```python
from build123d import *

# Parameters (mm, degrees)
SKETCH1_R           = 9.525
BOSS_EXTRUDE1_DEPTH = 6.35
CUT_EXTRUDE1_START  = -6.35
CUT_EXTRUDE1_DEPTH  = 6.35
CUT_EXTRUDE2_START  = -6.35
CUT_EXTRUDE2_DEPTH  = 6.35
SKETCH4_R           = 1.254125
CUT_EXTRUDE3_DEPTH  = 10.525
SKETCH4_3_R         = 1.254125
CUT_EXTRUDE4_DEPTH  = 10.5250001


with BuildPart() as part:
    # Sketch1 → Boss-Extrude1 (new body, symmetric)
    with BuildSketch(Plane(origin=(0, 0, 0), x_dir=(1, 0, 0), z_dir=(0, 1, 0))):
        Circle(SKETCH1_R)
    extrude(amount=BOSS_EXTRUDE1_DEPTH, both=True)

    # Sketch2 → Cut-Extrude1 (cut)
    with BuildSketch(Plane(origin=(0, 6.35, 0), x_dir=(1, 0, 0), z_dir=(0, 1, 0)).offset(CUT_EXTRUDE1_START)):
        with BuildLine():
            Line((1.8415, 1.840404847), (1.8415, -1.840404847))
            ThreePointArc((1.8415, -1.840404847), (-2.6035, 0), (1.8415, 1.840404847))
        make_face()
    extrude(amount=CUT_EXTRUDE1_DEPTH, mode=Mode.SUBTRACT)

    # Sketch3 → Cut-Extrude2 (cut)
    with BuildSketch(Plane.XZ.offset(6.35).offset(CUT_EXTRUDE2_START)):
        with BuildLine():
            Line((2.449999926, 3.224903191), (2.449999926, -3.224903191))
            ThreePointArc((2.449999926, -3.224903191), (-4.050000028, 0), (2.449999926, 3.224903191))
        make_face()
    extrude(amount=CUT_EXTRUDE2_DEPTH, mode=Mode.SUBTRACT)

    # Sketch4 → Cut-Extrude3 (cut, through all)
    with BuildSketch(Plane(origin=(0, 0, 0), x_dir=(0, 0, -1), z_dir=(1, 0, 0))):
        with Locations((0, -3.389153937)):
            Circle(SKETCH4_R)
    extrude(amount=-CUT_EXTRUDE3_DEPTH, mode=Mode.SUBTRACT)

    # Sketch4<3> → Cut-Extrude4 (cut, through all)
    with BuildSketch(Plane(origin=(0, 0, 0), x_dir=(0, 0, -1), z_dir=(1, 0, 0))):
        with Locations((0, 3.690412064)):
            Circle(SKETCH4_3_R)
    extrude(amount=CUT_EXTRUDE4_DEPTH, mode=Mode.SUBTRACT)


solid = part.part
```
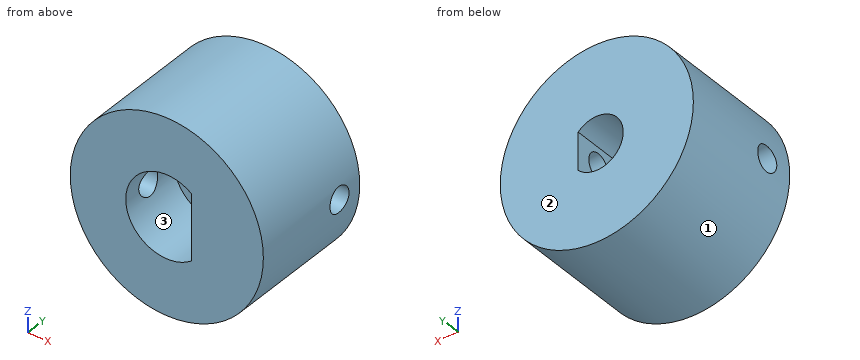
Geometry check sheet. Reference: the model listing, model coordinates, mm. Face numbers are marked on the shaded views. Round coordinates to 2 decimals unless told otherwise and drop trailing zeros. Write each loop counter-clockwise with the first axis right and the second up, starting at its lowest first coordinate (ties: lowest second). Pieces come first, ordered by that corner, then holes. Notation, with made-up numbers: (-12, 13) - (18, 13) arc R10 ccw to (18, 22) - close; hole circle Ø7 at (67.5, 28.5). An arc over 180 degrees is marked (long way). Write each question's results on one line, items separated by ' | '.
(1) Sectioned sample at D-D, the plane x = 6.5. Enter the section's corners in (y, z), plus the area to 3 significant figures.
Computed:
outline: (-6.35, -6.96) - (6.35, -6.96) - (6.35, 6.96) - (-6.35, 6.96) - close; hole circle Ø2.51 at (3.69, 0) | area: 172 mm^2
(2) Draft check along X on the marked faces 1, 2 and 3. Enter one of: pulls with the +X half, pulls with the -X half, needs draft (parallel to the pull), parting line crosses it, or undercut.
Computed:
face 1: parting line crosses it | face 2: needs draft | face 3: undercut
(3) Thickness scan on probe 1 along Y at (x, z) = (5.25, 0); probe 2 along Y at (x, z) = (-7.2, 0); probe 3 along X at (y, z) = (-1.25, 0) (3 decimals). Record the ranges inside material, lowest first. Write a range as from..to.
Computed:
probe 1: y = -6.35..2.44, 4.94..6.35 | probe 2: y = -6.35..-4.64, -2.14..6.35 | probe 3: x = -9.525..-4.05, 2.45..9.525
(4) Depth check by flat-ended pin: pin 1 Ø2 at (y, z) = (4, 1.5) entering from -X; pin 2 Ø1 at (y, z) = (-3.5, 4) entering from +X; pin 3 Ø6 at (y, z) = (-4.5, -7) entering from +X. Enter the tip coordinate at first touch or a pass-through.
Computed:
pin 1: stops at x = -9.51 | pin 2: stops at x = 8.86 | pin 3: stops at x = 8.64
(5) Sectioned sample at B-B, the plane z = 0. Count the separate pieces of the cut face and the enclosed holes in it, plus the area to 3 significant figures.
Computed:
separate pieces: 4 | enclosed holes: 0 | area: 139 mm^2
(6) Sectioned sample at C-C, the plane y = -0.5. Enter the section's corners in (x, z) (3 decimals), plus the area to 3 significant figures.
Computed:
outline: circle Ø19.05 at (0, 0); hole (2.45, -3.225) - (2.45, 3.225) arc R4.05 ccw (long way) to start | area: 241 mm^2
